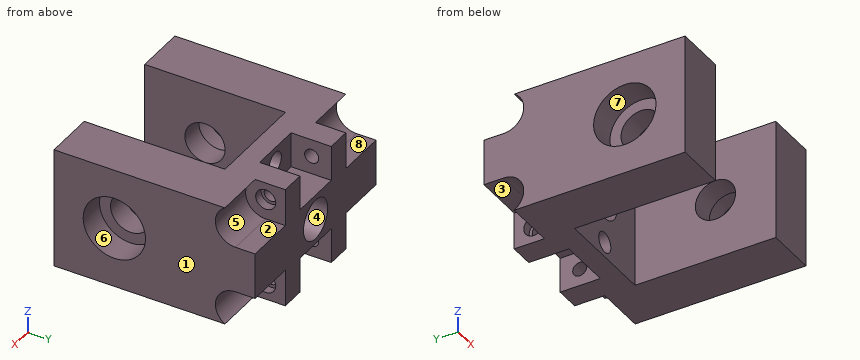
from build123d import *

# Parameters (mm, degrees)
SKETCH_1_W                = 10
SKETCH_1_H                = 12
EXTRUDE_1_DEPTH           = 6
SKETCH_2_R                = 1
CUT_EXTRUDE_1_DEPTH       = 17.733200531
SKETCH_2_3_R              = 2
CUT_EXTRUDE_2_DEPTH       = 4
SKETCH_3_R                = 2
CUT_EXTRUDE_3_DEPTH       = 17.733200531
SKETCH_4_W                = 5.2
SKETCH_4_H                = 3.5
CUT_EXTRUDE_4_DEPTH       = 4
SKETCH_6_R                = 0.7
CUT_EXTRUDE_5_DEPTH       = 17.733200531
SKETCH_6_3_R              = 1
CUT_EXTRUDE_6_DEPTH       = 0.9
CUT_EXTRUDE_START         = -9.1
SKETCH_6_4_R              = 1
CUT_EXTRUDE_7_DEPTH       = 0.9
SKETCH_7_W                = 12
SKETCH_7_H                = 20
EXTRUDE_2_DEPTH           = 5
CUT_EXTRUDE_START_2       = 5
CUT_EXTRUDE_8_DEPTH       = 5
EXTRUDE_START             = -10
SKETCH_7_4_W              = 12
SKETCH_7_4_H              = 20
EXTRUDE_3_DEPTH           = 5
CUT_EXTRUDE_START_3       = -10
SKETCH_7_5_R              = 1
CUT_EXTRUDE_9_DEPTH       = 5
CUT_EXTRUDE_10_DEPTH      = 24.769728648
CUT_EXTRUDE_10_DEPTH_BACK = 24.769728648
SKETCH_7_6_R              = 2
SKETCH_7_7_R              = 3.1
CUT_EXTRUDE_11_DEPTH      = 2.7
CUT_EXTRUDE_START_4       = -12.3
SKETCH_7_8_R              = 3.1
CUT_EXTRUDE_12_DEPTH      = 2.7


with BuildPart() as part:
    # 草图1 → 凸台-拉伸1 (new body)
    with BuildSketch(Plane(origin=(0, 0, 0), x_dir=(1, 0, 0), z_dir=(0, 1, 0))):
        with Locations((5, -6)):
            Rectangle(SKETCH_1_W, SKETCH_1_H)
    extrude(amount=EXTRUDE_1_DEPTH)

    # 草图2 → 切除-拉伸1 (cut, through all)
    with BuildSketch(Plane(origin=(0, 6, 0), x_dir=(1, 0, 0), z_dir=(0, 1, 0))):
        with Locations(Location((5, -1.5, 0), (0, 0, 270))):
            Circle(SKETCH_2_R)
        with Locations(Location((5, -10.5, 0), (0, 0, 270))):
            Circle(SKETCH_2_R)
    extrude(amount=-CUT_EXTRUDE_1_DEPTH, mode=Mode.SUBTRACT)

    # 草图2<3> → 切除-拉伸2 (cut)
    with BuildSketch(Plane(origin=(0, 6, 0), x_dir=(1, 0, 0), z_dir=(0, 1, 0))):
        with Locations((5, -1.5)):
            Circle(SKETCH_2_3_R)
        with Locations((5, -10.5)):
            Circle(SKETCH_2_3_R)
    extrude(amount=-CUT_EXTRUDE_2_DEPTH, mode=Mode.SUBTRACT)

    # 草图3 → 切除-拉伸3 (cut, through all)
    with BuildSketch(Plane(origin=(0, 6, 0), x_dir=(1, 0, 0), z_dir=(0, 1, 0))):
        with Locations(Location((5, -6, 0), (0, 0, 270))):
            Circle(SKETCH_3_R)
    extrude(amount=-CUT_EXTRUDE_3_DEPTH, mode=Mode.SUBTRACT)

    # 草图4 → 切除-拉伸4 (cut)
    with BuildSketch(Plane(origin=(0, 6, 0), x_dir=(1, 0, 0), z_dir=(0, 1, 0))):
        with Locations((5, -1.75)):
            Rectangle(SKETCH_4_W, SKETCH_4_H)
        with Locations((5, -10.25)):
            Rectangle(SKETCH_4_W, SKETCH_4_H)
    extrude(amount=-CUT_EXTRUDE_4_DEPTH, mode=Mode.SUBTRACT)

    # 草图6 → 切除-拉伸5 (cut, through all)
    with BuildSketch(Plane.ZY):
        with Locations((1.7, 4.05)):
            Circle(SKETCH_6_R)
        with Locations((10.3, 4.05)):
            Circle(SKETCH_6_R)
    extrude(amount=-CUT_EXTRUDE_5_DEPTH, mode=Mode.SUBTRACT)

    # 草图6<3> → 切除-拉伸6 (cut)
    with BuildSketch(Plane.ZY):
        with Locations((1.7, 4.05)):
            Circle(SKETCH_6_3_R)
        with Locations((10.3, 4.05)):
            Circle(SKETCH_6_3_R)
    extrude(amount=-CUT_EXTRUDE_6_DEPTH, mode=Mode.SUBTRACT)

    # 草图6<4> → 切除-拉伸7 (cut)
    with BuildSketch(Plane.ZY.offset(CUT_EXTRUDE_START)):
        with Locations((1.7, 4.05)):
            Circle(SKETCH_6_4_R)
        with Locations((10.3, 4.05)):
            Circle(SKETCH_6_4_R)
    extrude(amount=-CUT_EXTRUDE_7_DEPTH, mode=Mode.SUBTRACT)

    # 草图7 → 凸台-拉伸2 (add)
    with BuildSketch(Plane(origin=(10, 0, 0), x_dir=(0, 0, -1), z_dir=(1, 0, 0))):
        with Locations((-6, -4)):
            Rectangle(SKETCH_7_W, SKETCH_7_H)
    extrude(amount=EXTRUDE_2_DEPTH)

    # 草图7<3> → 切除-拉伸8 (cut)
    with BuildSketch(Plane(origin=(10, 0, 0), x_dir=(0, 0, -1), z_dir=(1, 0, 0)).offset(CUT_EXTRUDE_START_2)):
        with BuildLine():
            ThreePointArc((-8.3, 4.05), (-8.736539185, 5.297233049), (-9.855590279, 6))
            Line((-9.855590279, 6), (-10.744409721, 6))
            ThreePointArc((-10.744409721, 6), (-11.462119625, 5.677721714), (-12, 5.103565375))
            Line((-12, 5.103565375), (-12, 2.996434625))
            ThreePointArc((-12, 2.996434625), (-9.752277442, 2.126461594), (-8.3, 4.05))
        make_face()
        with BuildLine():
            ThreePointArc((-12, 5.103565375), (-11.462119625, 5.677721714), (-10.744409721, 6))
            Line((-10.744409721, 6), (-12, 6))
            Line((-12, 6), (-12, 5.103565375))
        make_face()
        with BuildLine():
            Line((-1.255590279, 6), (-2.144409721, 6))
            ThreePointArc((-2.144409721, 6), (-3.263460815, 5.297233049), (-3.7, 4.05))
            ThreePointArc((-3.7, 4.05), (-2.247722558, 2.126461594), (0, 2.996434625))
            Line((0, 2.996434625), (0, 5.103565375))
            ThreePointArc((0, 5.103565375), (-0.537880375, 5.677721714), (-1.255590279, 6))
        make_face()
        with BuildLine():
            Line((0, 6), (-1.255590279, 6))
            ThreePointArc((-1.255590279, 6), (-0.537880375, 5.677721714), (0, 5.103565375))
            Line((0, 5.103565375), (0, 6))
        make_face()
        with BuildLine():
            Line((-8.3, 4.05), (-8.3, 6))
            Line((-8.3, 6), (-9.855590279, 6))
            ThreePointArc((-9.855590279, 6), (-8.736539185, 5.297233049), (-8.3, 4.05))
        make_face()
        with BuildLine():
            Line((-2.144409721, 6), (-3.7, 6))
            Line((-3.7, 6), (-3.7, 4.05))
            ThreePointArc((-3.7, 4.05), (-3.263460815, 5.297233049), (-2.144409721, 6))
        make_face()
    extrude(amount=-CUT_EXTRUDE_8_DEPTH, mode=Mode.SUBTRACT)

    # 草图7<4> → 凸台-拉伸3 (add)
    with BuildSketch(Plane(origin=(10, 0, 0), x_dir=(0, 0, -1), z_dir=(1, 0, 0)).offset(EXTRUDE_START)):
        with Locations((-6, -4)):
            Rectangle(SKETCH_7_4_W, SKETCH_7_4_H)
    extrude(amount=-EXTRUDE_3_DEPTH)

    # 草图7<5> → 切除-拉伸9 (cut)
    # profile 1 of 8: a face of its own
    with BuildSketch(Plane(origin=(10, 0, 0), x_dir=(0, 0, -1), z_dir=(1, 0, 0)).offset(CUT_EXTRUDE_START_3)):
        with BuildLine():
            ThreePointArc((-8.3, 4.05), (-8.736539185, 5.297233049), (-9.855590279, 6))
            Line((-9.855590279, 6), (-10.744409721, 6))
            ThreePointArc((-10.744409721, 6), (-11.462119625, 5.677721714), (-12, 5.103565375))
            Line((-12, 5.103565375), (-12, 2.996434625))
            ThreePointArc((-12, 2.996434625), (-9.752277442, 2.126461594), (-8.3, 4.05))
        make_face()
        with Locations(Location((-10.3, 4.05, 0), (0, 0, 180))):
            Circle(SKETCH_7_5_R, mode=Mode.SUBTRACT)
    # profile 2 of 8: a face of its own
    with BuildSketch(Plane(origin=(10, 0, 0), x_dir=(0, 0, -1), z_dir=(1, 0, 0)).offset(CUT_EXTRUDE_START_3)):
        with BuildLine():
            Line((-8.3, 4.05), (-8.3, 6))
            Line((-8.3, 6), (-9.855590279, 6))
            ThreePointArc((-9.855590279, 6), (-8.736539185, 5.297233049), (-8.3, 4.05))
        make_face()
    # profile 3 of 8: a face of its own
    with BuildSketch(Plane(origin=(10, 0, 0), x_dir=(0, 0, -1), z_dir=(1, 0, 0)).offset(CUT_EXTRUDE_START_3)):
        with BuildLine():
            ThreePointArc((-12, 5.103565375), (-11.462119625, 5.677721714), (-10.744409721, 6))
            Line((-10.744409721, 6), (-12, 6))
            Line((-12, 6), (-12, 5.103565375))
        make_face()
    # profile 4 of 8: a face of its own
    with BuildSketch(Plane(origin=(10, 0, 0), x_dir=(0, 0, -1), z_dir=(1, 0, 0)).offset(CUT_EXTRUDE_START_3)):
        with BuildLine():
            Line((-1.255590279, 6), (-2.144409721, 6))
            ThreePointArc((-2.144409721, 6), (-3.263460815, 5.297233049), (-3.7, 4.05))
            ThreePointArc((-3.7, 4.05), (-2.247722558, 2.126461594), (0, 2.996434625))
            Line((0, 2.996434625), (0, 5.103565375))
            ThreePointArc((0, 5.103565375), (-0.537880375, 5.677721714), (-1.255590279, 6))
        make_face()
        with Locations(Location((-1.7, 4.05, 0), (0, 0, 180))):
            Circle(SKETCH_7_5_R, mode=Mode.SUBTRACT)
    # profile 5 of 8: a face of its own
    with BuildSketch(Plane(origin=(10, 0, 0), x_dir=(0, 0, -1), z_dir=(1, 0, 0)).offset(CUT_EXTRUDE_START_3)):
        with BuildLine():
            Line((-2.144409721, 6), (-3.7, 6))
            Line((-3.7, 6), (-3.7, 4.05))
            ThreePointArc((-3.7, 4.05), (-3.263460815, 5.297233049), (-2.144409721, 6))
        make_face()
    # profile 6 of 8: a face of its own
    with BuildSketch(Plane(origin=(10, 0, 0), x_dir=(0, 0, -1), z_dir=(1, 0, 0)).offset(CUT_EXTRUDE_START_3)):
        with BuildLine():
            Line((0, 6), (-1.255590279, 6))
            ThreePointArc((-1.255590279, 6), (-0.537880375, 5.677721714), (0, 5.103565375))
            Line((0, 5.103565375), (0, 6))
        make_face()
    # profile 7 of 8: a face of its own
    with BuildSketch(Plane(origin=(10, 0, 0), x_dir=(0, 0, -1), z_dir=(1, 0, 0)).offset(CUT_EXTRUDE_START_3)):
        with Locations(Location((-10.3, 4.05, 0), (0, 0, 180))):
            Circle(SKETCH_7_5_R)
    # profile 8 of 8: a face of its own
    with BuildSketch(Plane(origin=(10, 0, 0), x_dir=(0, 0, -1), z_dir=(1, 0, 0)).offset(CUT_EXTRUDE_START_3)):
        with Locations(Location((-1.7, 4.05, 0), (0, 0, 180))):
            Circle(SKETCH_7_5_R)
    extrude(amount=-CUT_EXTRUDE_9_DEPTH, mode=Mode.SUBTRACT)

    # 草图7<6> → 切除-拉伸10 (cut, two sides: drawn at the far end of the back side and taken through both)
    with BuildSketch(Plane(origin=(10, 0, 0), x_dir=(0, 0, -1), z_dir=(1, 0, 0)).offset(-CUT_EXTRUDE_10_DEPTH_BACK)):
        with Locations((-6, -8)):
            Circle(SKETCH_7_6_R)
    extrude(amount=CUT_EXTRUDE_10_DEPTH + CUT_EXTRUDE_10_DEPTH_BACK, mode=Mode.SUBTRACT)

    # 草图7<7> → 切除-拉伸11 (cut)
    with BuildSketch(Plane(origin=(10, 0, 0), x_dir=(0, 0, -1), z_dir=(1, 0, 0)).offset(CUT_EXTRUDE_START_2)):
        with Locations((-6, -8)):
            Circle(SKETCH_7_7_R)
    extrude(amount=-CUT_EXTRUDE_11_DEPTH, mode=Mode.SUBTRACT)

    # 草图7<8> → 切除-拉伸12 (cut)
    with BuildSketch(Plane(origin=(10, 0, 0), x_dir=(0, 0, -1), z_dir=(1, 0, 0)).offset(CUT_EXTRUDE_START_4)):
        with Locations((-6, -8)):
            Circle(SKETCH_7_8_R)
    extrude(amount=-CUT_EXTRUDE_12_DEPTH, mode=Mode.SUBTRACT)


solid = part.part
Design review of the part built by this model. Coordinates are the model's own, in mm. Face numbers are marked on the shaded views. A direction names the side the tool comes from. Coordinates: 2 decimals unless noted, no trailing zeros. Write each loop counter-clockwise with the first axis right and the second up, starting at its lowest first coordinate (ties: lowest second). Pieces come first, ordered by that corner, then holes. Notation, with made-up numbers: (-28.5, -16.75) - (10.5, -16.75) arc R32 cw to (10.5, 10.25) - close; hole circle Ø3 at (78.25, 81). An arc over 180 degrees is marked (long way). One line per item, written item: value.
1) Insertion check: pin 1 (1.6 mm diameter, centred on x = -1.5, y = 5.5, fed in from -Z); pin 2 (4 mm diameter, centred on y = 4.5, z = 10.5, fed in from +X); pin 3 (1.8 mm diameter, centred on y = 4.05, z = 10.3, fed in from -X). Each pin has a flat end and moves straight along its axis. Give the tip position at first contact, or say it passes through.
Answer sheet:
pin 1: stops at z = 3.7
pin 2: stops at x = 10
pin 3: stops at x = 0.9
2) For the marked faces 5, 6, 7 and 8, list the 3-axis set-ups (+Z, -Z, +X, -X, +Y, -Y) from which the entire face can be reached by the end or side of a thin tool; tool diameter is ignored.
Answer sheet:
face 5: +X, +Y
face 6: +X
face 7: -X
face 8: +Z, -X, +Y
3) Mouldability with a two-part tool opening along Z and no side actions: class the marked faces 1, 2, 3 and 4 as +Z half, -Z half, draft (parallel to the pull), parting line (faces both ways), or undercut.
Answer sheet:
face 1: draft
face 2: +Z half
face 3: -Z half
face 4: undercut
4) Add section D-D (x = 8.75). State the section outline as (y, z) points, plus the area to 3 significant figures.
Answer sheet:
outline: (0, 0) - (6, 0) - (6, 12) - (0, 12) - close; hole circle Ø1.4 at (4.05, 1.7); hole circle Ø1.4 at (4.05, 10.3)
area: 68.9 mm2
5) Add section C-C (y = -2.25). State the section outline as (x, z) points.
Answer sheet:
outline: (-5, 0) - (0, 0) - (0, 12) - (-5, 12) - close; (10, 0) - (15, 0) - (15, 12) - (10, 12) - close
6) Add section A-A (y = -8). State the section outline as (x, z) points, plus the area to 3 significant figures.
Answer sheet:
outline: (-5, 0) - (0, 0) - (0, 4) - (-2.3, 4) - (-2.3, 2.9) - (-5, 2.9) - close; (-5, 9.1) - (-2.3, 9.1) - (-2.3, 8) - (0, 8) - (0, 12) - (-5, 12) - close; (10, 0) - (15, 0) - (15, 2.9) - (12.3, 2.9) - (12.3, 4) - (10, 4) - close; (10, 8) - (12.3, 8) - (12.3, 9.1) - (15, 9.1) - (15, 12) - (10, 12) - close
area: 68.1 mm2
7) To check wall thickness, follow probe 1 along X at (y, z) = (4.75, 9); probe 2 along Y at (x, z) = (-3.55, 6); probe 3 along X at (y, z) = (-10, 9). State the ranges of each line that lie inside material, in increasing order.
Answer sheet:
probe 1: x = 0 to 2.4, 7.6 to 10
probe 2: y = -14 to -11.1, -4.9 to 6
probe 3: x = -5 to 0, 10 to 15
8) Add section B-B (z = 6). State the section outline as (x, y) points.
Answer sheet:
outline: (-5, -14) - (0, -14) - (0, -10) - (-2.3, -10) - (-2.3, -11.1) - (-5, -11.1) - close; (-5, -4.9) - (-2.3, -4.9) - (-2.3, -6) - (0, -6) - (0, 0) - (3, 0) - (3, 6) - (-5, 6) - close; (7, 0) - (10, 0) - (10, -6) - (12.3, -6) - (12.3, -4.9) - (15, -4.9) - (15, 6) - (7, 6) - close; (10, -14) - (15, -14) - (15, -11.1) - (12.3, -11.1) - (12.3, -10) - (10, -10) - close
